Could you check a few things on this model? Use its own coordinates, in mm. Face numbers are marked on the shaded views. A direction names the side the tool comes from. Give positions to 0.01 mm unless a question says otherwise; leave off trailing zeros. Write each loop counter-clockwise with the first axis right and the second up, starting at its lowest first coordinate (ties: lowest second). Pieces come first, ordered by that corner, then holes. Notation, with made-up numbers: M 14,-24.75 L 71,-24.75 A18 cw 71,-14.75 Z; hole C 31.25,-28 d11. An arc over 180 degrees is marked long. One line per item, written item: value.
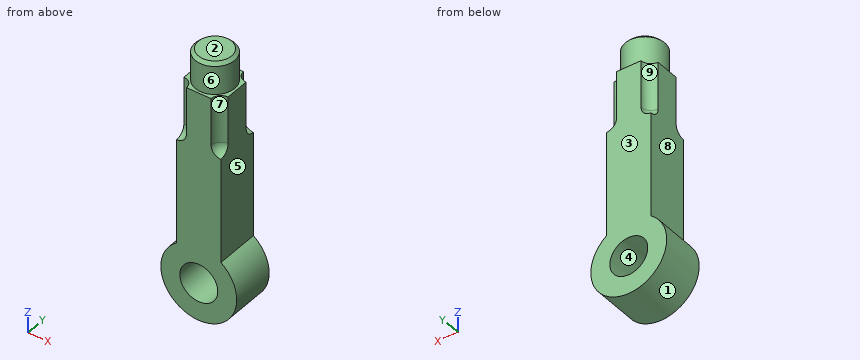
```python
from build123d import *

# Parameters (mm, degrees)
SKETCH1_R           = 24
SKETCH1_R_2         = 12
BOSS_EXTRUDE1_DEPTH = 14
BOSS_EXTRUDE2_REACH = 148
SKETCH2_W           = 28
SKETCH2_H           = 28
SKETCH4_R           = 12.5
BOSS_EXTRUDE3_DEPTH = 20
CHAMFER1_SIZE       = 2


with BuildPart() as part:
    # Sketch1 → Boss-Extrude1 (new body, symmetric)
    with BuildSketch(Plane(origin=(0, 0, 0), x_dir=(1, 0, 0), z_dir=(0, 1, 0))):
        Circle(SKETCH1_R)
        Circle(SKETCH1_R_2, mode=Mode.SUBTRACT)
    extrude(amount=BOSS_EXTRUDE1_DEPTH, both=True)

    # Sketch2 → Boss-Extrude2 (add, up to next)
    with BuildSketch(Plane.XY.offset(122), mode=Mode.PRIVATE) as boss_extrude2_sk1:
        Rectangle(SKETCH2_W, SKETCH2_H)
    boss_extrude2_tool1 = extrude(boss_extrude2_sk1.sketch, amount=-BOSS_EXTRUDE2_REACH, mode=Mode.PRIVATE) - part.part
    add(boss_extrude2_tool1.solids().sort_by_distance((0, 0, 122))[0])

    # Sketch3 → Cut-Revolve1 (revolve, cut)
    with BuildSketch(Plane(origin=(14, 0, 0), x_dir=(0, 0, -1), z_dir=(1, 0, 0))):
        with BuildLine():
            Line((-122, 14), (-122, 7.78))
            Line((-122, 7.78), (-92, 7.78))
            ThreePointArc((-92, 7.78), (-87.601795821, 9.601795821), (-85.78, 14))
            Line((-85.78, 14), (-122, 14))
        make_face()
    cut_revolve1 = revolve(axis=Axis((14, 14, -500000), (0, 0, 1)), mode=Mode.SUBTRACT)

    # Mirror1: Cut-Revolve1 across plane
    add(cut_revolve1.mirror(Plane(origin=(0, 0, 0), x_dir=(0, 0, 1), z_dir=(1, 0, 0))), mode=Mode.SUBTRACT)

    # Mirror2: Cut-Revolve1 across plane
    add(cut_revolve1.mirror(Plane.ZX), mode=Mode.SUBTRACT)

    # Mirror2 copy 1 sketch → Mirror2 copy 1 (revolve, cut)
    with BuildSketch(Plane(origin=(-14, 0, 0), x_dir=(0, 0, -1), z_dir=(-1, 0, 0))):
        with BuildLine():
            Line((-122, 14), (-122, 7.78))
            Line((-122, 7.78), (-92, 7.78))
            ThreePointArc((-92, 7.78), (-87.601795821, 9.601795821), (-85.78, 14))
            Line((-85.78, 14), (-122, 14))
        make_face()
    revolve(axis=Axis((-14, -14, -500000), (0, 0, 1)), mode=Mode.SUBTRACT)

    # Sketch4 → Boss-Extrude3 (add)
    with BuildSketch(Plane.XY.offset(122)):
        Circle(SKETCH4_R)
    extrude(amount=BOSS_EXTRUDE3_DEPTH)

    # Chamfer1
    chamfer1_edges = [part.edges().sort_by_distance(p)[0] for p in [
        (-12.5, 0, 142),
    ]]
    chamfer(chamfer1_edges, length=CHAMFER1_SIZE)


solid = part.part
```
1) I'm going to push flat-ended pins straight in: pin 1 (5 mm diameter, centred on x = 13.5, y = -3.5, fed in from +Z); pin 2 (12 mm diameter, centred on x = 9.5, y = 6.5, fed in from -Z); pin 3 (2 mm diameter, centred on y = -4.5, z = 117, fed in from -X); pin 4 (21.5 mm diameter, centred on x = 0, z = 0, fed in from +Y). Where does each tip first touch, or does it pass through?
Outcome:
pin 1: stops at z = 141.05
pin 2: stops at z = -23.74
pin 3: stops at x = -14
pin 4: passes through
2) If we section it at C-C, the plane y = 0: Write out the boundary of the cut face in (x, z).
Outcome:
outline: M -14,19.49 A24 ccw long 14,19.49 L 14,122 L 12.5,122 L 12.5,140 L 10.5,142 L -10.5,142 L -12.5,140 L -12.5,122 L -14,122 Z; hole C 0,0 d24
3) If we section it at D-D, the plane z = 59.5: Write out the boundary of the cut face in (x, y), then the cut area to 3 significant figures.
Outcome:
outline: M -14,-14 L 14,-14 L 14,14 L -14,14 Z
area: 784 mm^2
4) We'd pull the mould along Z, two halves only. Please class the marked faces 1, 2, 3 and 4: pulls with the +Z half, pulls with the -Z half, needs draft (parallel to the pull), parting line crosses it, or undercut.
Outcome:
face 1: parting line crosses it
face 2: pulls with the +Z half
face 3: needs draft
face 4: undercut
5) If we section it at A-A, the plane x = 0: Write out the boundary of the cut face in (y, z), then the cut area to 3 significant figures.
Outcome:
outline: M -14,-24 L 14,-24 L 14,-12 L -14,-12 Z; M -14,12 L 14,12 L 14,122 L 12.5,122 L 12.5,140 L 10.5,142 L -10.5,142 L -12.5,140 L -12.5,122 L -14,122 Z
area: 3,910 mm^2
6) On a 3-axis mill with a long thin cutter (end or side, diameter ignored), from which of +Z, -Z, +X, -X, +Y, -Y can I reach the whole of each face in a straight line? I mean the marked faces 5, 6, 7, 8 and 9. Say none if no direction works.
Outcome:
face 5: +Z, +X, +Y, -Y
face 6: +Z
face 7: +Z, +X, -Y
face 8: +Z, -X, +Y, -Y
face 9: +Z, -X, +Y
7) Please list where these lines run through material, in increasing order: L1, parallel to X at y = -1.75, z = 0; L2, parallel to Z at x = -19.5, y = -11.75; L3, parallel to Z at x = 2.5, y = 12. Write a range as from..to.
Outcome:
L1: x = -24..-12, 12..24
L2: z = -13.99..13.99
L3: z = -23.87..-11.74, 11.74..140.24
8) If we section it at B-B, the plane z = 0: Write out the boundary of the cut face in (x, y).
Outcome:
outline: M -24,-14 L -12,-14 L -12,14 L -24,14 Z; M 12,-14 L 24,-14 L 24,14 L 12,14 Z
